Could you check a few things on this drawing? It's one solid part, dimensions in mm from its lowest x, y, z. A direction names the side the tool comes from. Round coordinates to 2 decimals unless told otherwise and drop trailing zeros. Write each loop counter-clockwise with the first axis right and the second up, starting at its lowest first coordinate (ties: lowest second). Pieces come first, ordered by that corner, then holes. Notation, with made-up numbers: (38, 16.25) -> (91, 16.25) arc R17 ccw to (91, 25.25) -> close; hole circle Ø5 at (13, 66). An arc over 180 degrees is marked (long way). Put each result on its own line as item: value. Start each with the question number.
1) I want a section at A-A, the plane x = 63.5. Give the number of separate pieces and of enclosed holes in the cut face, then the cut area to 3 significant figures.
2) If I drill on line 1 along Z through (x, y) = (63.5, 37.25) (1 decimal); line 2 along Y through (x, z) = (92, 38.5); line 3 along Z through (x, y) = (119, 22), over which ranges is the centre line in solid material (lowest first)? Write a range as [from, to].
3) I want a section at D-D, the plane z = 58. List the corners of the cut face in (x, y) for me.
4) We'd pull the mould along Y, two halves only. Please class the marked faces 1, 2 and 3: released by +Y, released by -Y, zero draft, split by the parting line, or undercut.
5) Which directions (+Z, -Z, +X, -X, +Y, -Y) give clear straight access to the entire face, cutting with the end or side of a thin tool? Please do the marked faces 4 and 5.
6) Will these pins go through, and if not, where does the flat tip stop? P1, Ø5, axis at y = 32, z = 39, coming from the +X side; P2, Ø1.5, axis at x = 61.5, y = 26.5, coming from the +Z side (1 decimal); P3, Ø1.9, axis at x = 56, y = 4.5, coming from the +Z side.
7) I want a section at B-B, the plane z = 18. List the corners of the cut face in (x, y) for me, then the cut area to 3 significant figures.
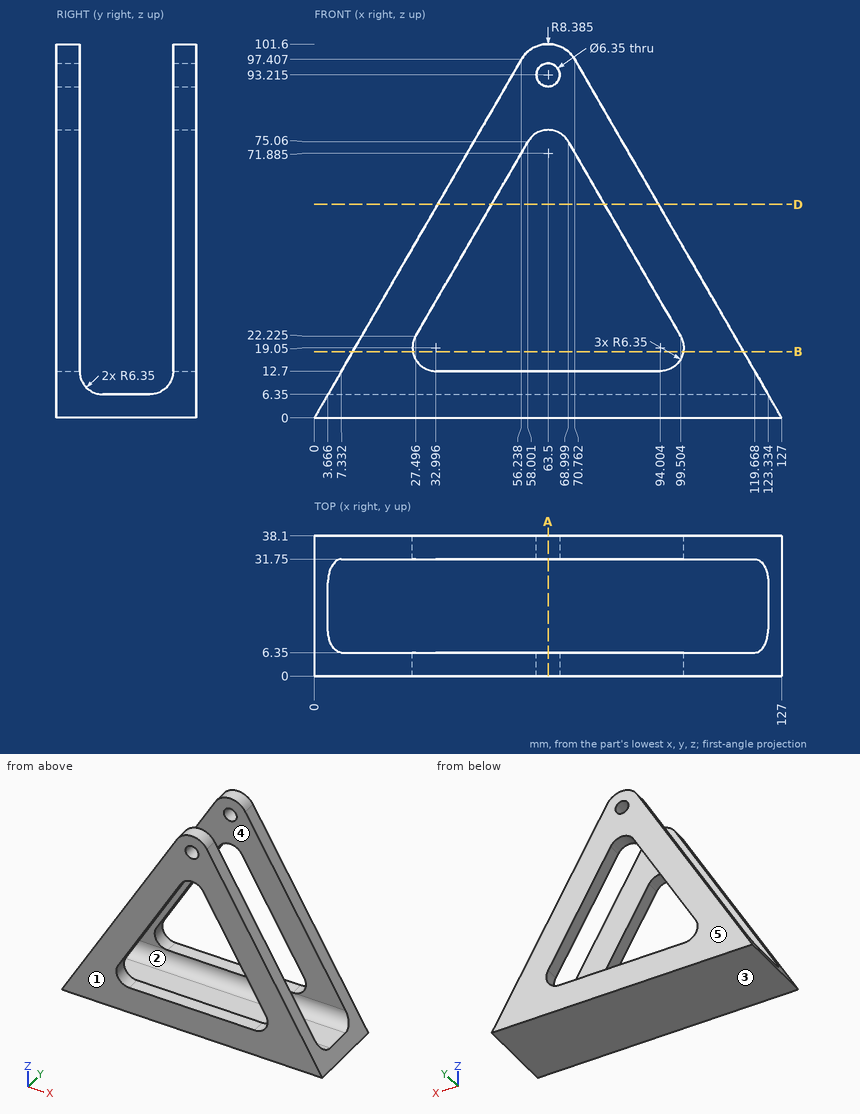
Findings:
1. separate pieces: 5
1. enclosed holes: 0
1. area: 556 mm2
2. line 1: z = [0, 12.7], [78.2, 90], [96.4, 101.6]
2. line 2: y = [0, 6.35], [31.75, 38.1]
2. line 3: z = [0, 6.35]
3. outline: (33.49, 0) -> (48.15, 0) -> (48.15, 6.35) -> (33.49, 6.35) -> close; (33.49, 31.75) -> (48.15, 31.75) -> (48.15, 38.1) -> (33.49, 38.1) -> close; (78.85, 0) -> (93.51, 0) -> (93.51, 6.35) -> (78.85, 6.35) -> close; (78.85, 31.75) -> (93.51, 31.75) -> (93.51, 38.1) -> (78.85, 38.1) -> close
4. face 1: released by -Y
4. face 2: undercut
4. face 3: zero draft
5. face 4: +Z, +X, -X
5. face 5: +Z, -Z, +X, -X, +Y
6. P1: stops at x = 105.93
6. P2: stops at z = 6.6
6. P3: stops at z = 98.45
7. outline: (10.39, 0) -> (26.73, 0) -> (26.73, 6.35) -> (10.39, 6.35) -> close; (10.39, 31.75) -> (26.73, 31.75) -> (26.73, 38.1) -> (10.39, 38.1) -> close; (100.27, 0) -> (116.61, 0) -> (116.61, 6.35) -> (100.27, 6.35) -> close; (100.27, 31.75) -> (116.61, 31.75) -> (116.61, 38.1) -> (100.27, 38.1) -> close
7. area: 415 mm2
